CAD build for the part. Positions are in the model's coordinates, mm. A direction names the side the tool comes from. Round coordinates to 2 decimals unless told otherwise and drop trailing zeros. Write each loop counter-clockwise with the first axis right and the second up, starting at its lowest first coordinate (ties: lowest second). Pieces come first, ordered by that corner, then holes. Notation, with made-up numbers: (79.5, 78.25) - (115.5, 78.25) arc R26 ccw to (115.5, 107.25) - close; hole circle Ø10 at (64, 36). An arc over 180 degrees is marked (long way). Put each result on its own line as item: value. Start each with the question number.
Item 1: 3-axis set-ups, long thin cutter, end or side, ignore diameter. For faces 4 (the flat face through (39, 0, -3)), 5 (the cylindrical face through (40.1, 0.39, -1.43)): which of +Z, -Z, +X, -X, +Y, -Y reach the whole face in a straight line?
Item 2: Mould opens along X. For faces 1 (the cylindrical face through (-0.727, -15.456, 18.89)), 2 (the flat face through (19, -5, 38.2)), 3 (the cylindrical face through (16.383, 0.134, 18.637)) say: released by +X, released by -X, zero draft, split by the parting line, or undercut.
Item 3: Cut at B-B (z = 15). Give the cut face in (x, y), and give its area (3 significant figures).
Item 4: Pin check, flat tips, straight feed: pin 1 Ø1 at (y, z) = (18, 29.5) entering from -X; pin 2 Ø5 at (y, z) = (-19.5, 14.5) entering from -X; pin 3 Ø15 at (x, y) = (11, -1.5) entering from -Z; pin 4 Ø5.5 at (x, y) = (19.43, 0) entering from +Z. Stop position of each tip, or through.
Item 5: Cut at A-A (x = 19.43). Give the cut face in (y, z), and give its area (3 significant figures).
Item 6: Drill centre lines: line 1 (Y direction, x = 19.43, z = 23); line 2 (Z direction, x = 1, y = 6); line 3 (Y direction, x = 27, z = 23.5). Where is each one in solid material? Low to high. Write a range as from..to.
```python
from build123d import *

# Parameters (mm, degrees)
SKETCH_R          = 25.4
SKETCH_R_2        = 3.05
PAD_DEPTH         = 38.1
FILLET_R          = 0.5
SKETCH001_R       = 1.3
PAD001_DEPTH      = 19.05
PAD001_DEPTH_BACK = 3.5


with BuildPart() as fillet_body:
    # Sketch → Pad (new body)
    with BuildSketch(Plane.XY.offset(0.1)):
        with Locations((19.43, 0)):
            Circle(SKETCH_R)
        with Locations((19.43, 0)):
            Circle(SKETCH_R_2, mode=Mode.SUBTRACT)
    extrude(amount=PAD_DEPTH)

    # Fillet
    fillet_edges = [fillet_body.edges().sort_by_distance(p)[0] for p in [
        (16.38, 0, 38.2),
        (-5.97, 0, 38.2),
        (-5.97, 0, 0.1),
    ]]
    fillet(fillet_edges, radius=FILLET_R)


with BuildPart() as obj1:
    # Sketch001 → Pad001 (new body, two sides)
    with BuildSketch(Plane.XY.offset(0.5)) as pad001_sk:
        Circle(SKETCH001_R)
        with Locations((38.86, 0)):
            Circle(SKETCH001_R)
    extrude(amount=PAD001_DEPTH)
    extrude(pad001_sk.sketch, amount=-PAD001_DEPTH_BACK)

    # obj1: union Fillet body
    add(fillet_body.part)


solid = obj1.part
```
Output values:
1. face 4: -Z, +X, -X, +Y, -Y
1. face 5: -Z
2. face 1: split by the parting line
2. face 2: zero draft
2. face 3: undercut
3. outline: circle Ø50.8 at (19.43, 0); hole circle Ø6.1 at (19.43, 0)
3. area: 2,000 mm2
4. pin 1: x = 1.02
4. pin 2: x = 0.56
4. pin 3: z = 0.1
4. pin 4: through
5. outline: (-25.4, 0.6) arc R0.5 ccw to (-24.9, 0.1) - (-3.05, 0.1) - (-3.05, 37.7) arc R0.5 ccw to (-3.55, 38.2) - (-24.9, 38.2) arc R0.5 ccw to (-25.4, 37.7) - close; (3.05, 0.1) - (24.9, 0.1) arc R0.5 ccw to (25.4, 0.6) - (25.4, 37.7) arc R0.5 ccw to (24.9, 38.2) - (3.55, 38.2) arc R0.5 ccw to (3.05, 37.7) - close
5. area: 1,700 mm2
6. line 1: -25.4..-3.05, 3.05..25.4
6. line 2: 0.1..38.2
6. line 3: -24.25..24.25
